Geometry check sheet. Reference: the model listing, model coordinates, mm. Round coordinates to 2 decimals unless told otherwise and drop trailing zeros. Order: outer loops, then holes, each group sorted by start corner. A loop starts at its lowest first (then second) coordinate and runs counter-clockwise, first axis right, second up.
(1) Sectioned sample at B-B (x = 270). Record the boundary of the cut face in (y, z), plus the area to 3 significant figures.
(2) Sectioned sample at A-A (x = 156.5). Record the boundary of the cut face in (y, z), plus the area to 3 significant figures.
(3) Material ranges on line 1 along Y through (x, z) = (270, 3.25); line 2 along Y through (x, z) = (178.5, 3.5), recorded low to high.
(4) Sectioned sample at C-C (y = 80). Record the boundary of the cut face in (x, z), plus the area to 3 significant figures.
(5) Sectioned sample at D-D (y = 59). Give the number of separate pieces and of enclosed holes in the cut face, plus the area to 3 significant figures.
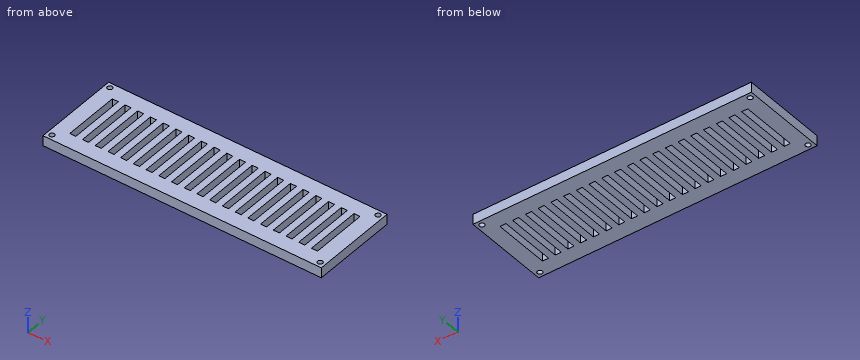
Autodesk Inventor part; units mm, degrees
ref_plane "YZ Plane" through (0, 0, 0) normal (1, 0, 0) x (0, 1, 0)
ref_plane "XZ Plane" through (0, 0, 0) normal (0, 1, 0) x (-1, 0, 0)
ref_plane "XY Plane" through (0, 0, 0) normal (0, 0, 1) x (1, 0, 0)
sketch "Sketch1" plane through (0, 0, 0) normal (0, 0, 1) x (1, 0, 0)
  line L0 (0, 0) -> (275, 0)
  line L1 (275, 0) -> (275, 85)
  line L2 (275, 85) -> (0, 85)
  line L3 (0, 85) -> (0, 0)
  dimension "d0" = 275
  dimension "d1" = 85
extrude "Extrusion1" add sketch "Sketch1" along normal blind 10
sketch "Sketch2" plane through (0, 0, 10) normal (0, 0, 1) x (1, 0, 0)
  line L0 (0, 0) -> (275, 0) construction
  line L1 (275, 0) -> (275, 85) construction
  line L2 (275, 85) -> (0, 85) construction
  line L3 (0, 85) -> (0, 0) construction
  line L4 (5, 80) -> (270, 80) construction
  line L5 (270, 80) -> (270, 5) construction
  line L6 (270, 5) -> (5, 5) construction
  line L7 (5, 5) -> (5, 80) construction
  line L8 (10, 75) -> (265, 75) construction
  line L9 (265, 75) -> (265, 10) construction
  line L10 (265, 10) -> (10, 10) construction
  line L11 (10, 10) -> (10, 75) construction
  circle A0 centre (5, 80) radius 2.5
  circle A1 centre (270, 80) radius 2.5
  circle A2 centre (270, 5) radius 2.5
  circle A3 centre (5, 5) radius 2.5
  line L12 (15, 70) -> (21, 70)
  line L13 (21, 70) -> (21, 15)
  line L14 (21, 15) -> (15, 15)
  line L15 (15, 15) -> (15, 70)
  line L16 (15, 70) -> (260, 70) construction
  line L17 (260, 70) -> (260, 15) construction
  line L18 (260, 15) -> (15, 15) construction
  line L19 (15, 15) -> (15, 70) construction
  line L20 (33.57, 70) -> (33.57, 15)
  line L21 (27.57, 70) -> (33.57, 70)
  line L22 (27.57, 15) -> (27.57, 70)
  line L23 (27.57, 15) -> (27.57, 70) construction
  line L24 (33.57, 15) -> (27.57, 15)
  line L25 (46.14, 70) -> (46.14, 15)
  line L26 (40.14, 70) -> (46.14, 70)
  line L27 (40.14, 15) -> (40.14, 70)
  line L28 (40.14, 15) -> (40.14, 70) construction
  line L29 (46.14, 15) -> (40.14, 15)
  line L30 (58.71, 70) -> (58.71, 15)
  line L31 (52.71, 70) -> (58.71, 70)
  line L32 (52.71, 15) -> (52.71, 70)
  line L33 (52.71, 15) -> (52.71, 70) construction
  line L34 (58.71, 15) -> (52.71, 15)
  line L35 (71.28, 70) -> (71.28, 15)
  line L36 (65.28, 70) -> (71.28, 70)
  line L37 (65.28, 15) -> (65.28, 70)
  line L38 (65.28, 15) -> (65.28, 70) construction
  line L39 (71.28, 15) -> (65.28, 15)
  line L40 (83.85, 70) -> (83.85, 15)
  line L41 (77.85, 70) -> (83.85, 70)
  line L42 (77.85, 15) -> (77.85, 70)
  line L43 (77.85, 15) -> (77.85, 70) construction
  line L44 (83.85, 15) -> (77.85, 15)
  line L45 (96.42, 70) -> (96.42, 15)
  line L46 (90.42, 70) -> (96.42, 70)
  line L47 (90.42, 15) -> (90.42, 70)
  line L48 (90.42, 15) -> (90.42, 70) construction
  line L49 (96.42, 15) -> (90.42, 15)
  line L50 (108.99, 70) -> (108.99, 15)
  line L51 (102.99, 70) -> (108.99, 70)
  line L52 (102.99, 15) -> (102.99, 70)
  line L53 (102.99, 15) -> (102.99, 70) construction
  line L54 (108.99, 15) -> (102.99, 15)
  line L55 (121.56, 70) -> (121.56, 15)
  line L56 (115.56, 70) -> (121.56, 70)
  line L57 (115.56, 15) -> (115.56, 70)
  line L58 (115.56, 15) -> (115.56, 70) construction
  line L59 (121.56, 15) -> (115.56, 15)
  line L60 (134.13, 70) -> (134.13, 15)
  line L61 (128.13, 70) -> (134.13, 70)
  line L62 (128.13, 15) -> (128.13, 70)
  line L63 (128.13, 15) -> (128.13, 70) construction
  line L64 (134.13, 15) -> (128.13, 15)
  line L65 (146.7, 70) -> (146.7, 15)
  line L66 (140.7, 70) -> (146.7, 70)
  line L67 (140.7, 15) -> (140.7, 70)
  line L68 (140.7, 15) -> (140.7, 70) construction
  line L69 (146.7, 15) -> (140.7, 15)
  line L70 (159.27, 70) -> (159.27, 15)
  line L71 (153.27, 70) -> (159.27, 70)
  line L72 (153.27, 15) -> (153.27, 70)
  line L73 (153.27, 15) -> (153.27, 70) construction
  line L74 (159.27, 15) -> (153.27, 15)
  line L75 (171.84, 70) -> (171.84, 15)
  line L76 (165.84, 70) -> (171.84, 70)
  line L77 (165.84, 15) -> (165.84, 70)
  line L78 (165.84, 15) -> (165.84, 70) construction
  line L79 (171.84, 15) -> (165.84, 15)
  line L80 (184.41, 70) -> (184.41, 15)
  line L81 (178.41, 70) -> (184.41, 70)
  line L82 (178.41, 15) -> (178.41, 70)
  line L83 (178.41, 15) -> (178.41, 70) construction
  line L84 (184.41, 15) -> (178.41, 15)
  line L85 (196.98, 70) -> (196.98, 15)
  line L86 (190.98, 70) -> (196.98, 70)
  line L87 (190.98, 15) -> (190.98, 70)
  line L88 (190.98, 15) -> (190.98, 70) construction
  line L89 (196.98, 15) -> (190.98, 15)
  line L90 (209.55, 70) -> (209.55, 15)
  line L91 (203.55, 70) -> (209.55, 70)
  line L92 (203.55, 15) -> (203.55, 70)
  line L93 (203.55, 15) -> (203.55, 70) construction
  line L94 (209.55, 15) -> (203.55, 15)
  line L95 (222.12, 70) -> (222.12, 15)
  line L96 (216.12, 70) -> (222.12, 70)
  line L97 (216.12, 15) -> (216.12, 70)
  line L98 (216.12, 15) -> (216.12, 70) construction
  line L99 (222.12, 15) -> (216.12, 15)
  line L100 (234.69, 70) -> (234.69, 15)
  line L101 (228.69, 70) -> (234.69, 70)
  line L102 (228.69, 15) -> (228.69, 70)
  line L103 (228.69, 15) -> (228.69, 70) construction
  line L104 (234.69, 15) -> (228.69, 15)
  line L105 (247.26, 70) -> (247.26, 15)
  line L106 (241.26, 70) -> (247.26, 70)
  line L107 (241.26, 15) -> (241.26, 70)
  line L108 (241.26, 15) -> (241.26, 70) construction
  line L109 (247.26, 15) -> (241.26, 15)
  line L110 (259.83, 70) -> (259.83, 15)
  line L111 (253.83, 70) -> (259.83, 70)
  line L112 (253.83, 15) -> (253.83, 70)
  line L113 (253.83, 15) -> (253.83, 70) construction
  line L114 (259.83, 15) -> (253.83, 15)
  dimension "d4" = 5
  dimension "d5" = 10
  dimension "d6" = 5
  dimension "d7" = 5
  dimension "d8" = 5
  dimension "d9" = 5
  dimension "d10" = 6
  dimension "d11" = 15
  dimension "d14" = 12.57
extrude "Extrusion2" cut sketch "Sketch2" against normal through all
properties part number "HA006" material "ABS Plastic"
Answer below:
1. outline: (0, 0) - (2.5, 0) - (2.5, 10) - (0, 10) - close; (7.5, 0) - (77.5, 0) - (77.5, 10) - (7.5, 10) - close; (82.5, 0) - (85, 0) - (85, 10) - (82.5, 10) - close
1. area: 750 mm2
2. outline: (0, 0) - (15, 0) - (15, 10) - (0, 10) - close; (70, 0) - (85, 0) - (85, 10) - (70, 10) - close
2. area: 300 mm2
3. line 1: y = 0 to 2.5, 7.5 to 77.5, 82.5 to 85
3. line 2: y = 0 to 15, 70 to 85
4. outline: (0, 0) - (2.5, 0) - (2.5, 10) - (0, 10) - close; (7.5, 0) - (267.5, 0) - (267.5, 10) - (7.5, 10) - close; (272.5, 0) - (275, 0) - (275, 10) - (272.5, 10) - close
4. area: 2,650 mm2
5. separate pieces: 21
5. enclosed holes: 0
5. area: 1,550 mm2
